Geometry check sheet. Reference: the model listing, model coordinates, mm. Coordinates: 2 decimals unless noted, no trailing zeros. Write each loop counter-clockwise with the first axis right and the second up, starting at its lowest first coordinate (ties: lowest second). Pieces come first, ordered by that corner, then holes. Notation, with made-up numbers: (71.25, 35) -> (93.25, 35) arc R14 cw to (93.25, 45) -> close; hole circle Ø6 at (-16.75, -39). An arc over 180 degrees is marked (long way). Use a Markdown table: item, result.
```python
from build123d import *

# Parameters (mm, degrees)
EXTRUDE_1_DEPTH = 1500
EXTRUDE_2_DEPTH = 50
EXTRUDE_5_DEPTH = 50
EXTRUDE_6_DEPTH = 50


with BuildPart() as part:
    # 草图2 → 拉伸-薄壁1 (new body)
    with BuildSketch(Plane.XY):
        Polygon((-2057.941251584, 400), (-457.941251584, 0), (-460.366607835, -9.701425001), (-2060.366607835, 390.298574999), align=None)
    extrude(amount=EXTRUDE_1_DEPTH)

    # 草图3 → 凸台-拉伸2 (add)
    with BuildSketch(Plane.XY.offset(1500)):
        Polygon((-1778.296514005, 330.088815605), (-1780.721870255, 320.387390604), (-1711.309316368, 303.034252132), (-1708.883960117, 312.735677133), align=None)
    extrude(amount=EXTRUDE_2_DEPTH)

    # 草图8 → 凸台-拉伸5 (add)
    with BuildSketch(Plane.XY.offset(1500)):
        Polygon((-841.962523584, 95.770350875), (-844.387879834, 86.068925873), (-774.975325947, 68.715787402), (-772.549969697, 78.417212403), align=None)
    extrude(amount=EXTRUDE_5_DEPTH)

    # 草图9 → 凸台-拉伸6 (add)
    with BuildSketch(Plane.XY.offset(1500)):
        Polygon((-1211.830765034, 187.137147041), (-1214.256121285, 177.435722039), (-1144.843567398, 160.082583568), (-1142.418211147, 169.784008569), align=None)
    extrude(amount=EXTRUDE_6_DEPTH)


solid = part.part
```
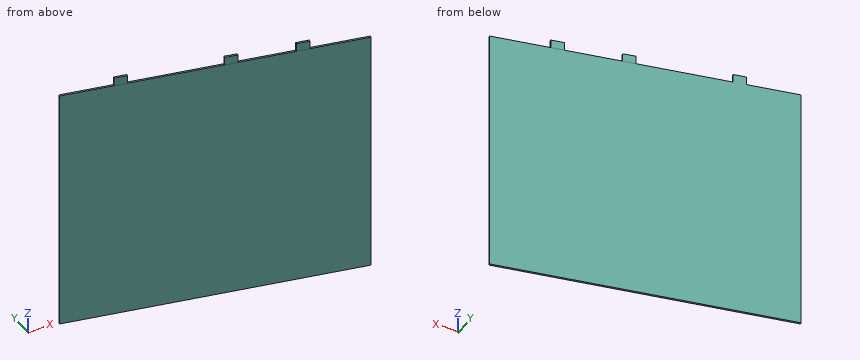
Item 1: Section check A-A on z = 653. Record the boundary of the cut face in (x, y).
Answer block:
| item | result |
|---|---|
| outline | (-2060.37, 390.3) -> (-460.37, -9.7) -> (-457.94, 0) -> (-2057.94, 400) -> close |
Item 2: Thickness scan on L1, parallel to Y at x = -930.5, z = 886.5; L2, parallel to Y at x = -1826, z = 1100. Record the ranges inside material, lowest first. Write a range as [from, to].
Answer block:
| item | result |
|---|---|
| L1 | y = [107.83, 118.14] |
| L2 | y = [331.71, 342.01] |
Item 3: Section check B-B on x = -1734. Record the boundary of the cut face in (y, z), then the cut area to 3 significant figures.
Answer block:
| item | result |
|---|---|
| outline | (308.71, 0) -> (319.01, 0) -> (319.01, 1550) -> (308.71, 1550) -> close |
| area | 16,000 mm^2 |
Item 4: Depth check by flat-ended pin: P1, Ø3, axis at x = -1004.5, z = 809, coming from the +Y side; P2, Ø1.5, axis at x = -809.5, z = 687, coming from the -Y side; P3, Ø3, axis at x = -1025, z = 312.5, coming from the -Y side. Enter the tip coordinate at first touch or a pass-through.
Answer block:
| item | result |
|---|---|
| P1 | stops at y = 137.01 |
| P2 | stops at y = 77.39 |
| P3 | stops at y = 131.08 |
